Build history of the part. All positions in model axes, mm. A direction names the side the tool comes from. Coordinates: 2 decimals unless noted, no trailing zeros. Write each loop counter-clockwise with the first axis right and the second up, starting at its lowest first coordinate (ties: lowest second). Pieces come first, ordered by that corner, then holes. Notation, with made-up numbers: (-34, -2.75) -> (17, -2.75) arc R21 ccw to (17, 10.25) -> close; hole circle Ø10 at (-6.75, 24). An arc over 180 degrees is marked (long way). Write each question's results on one line, items separated by ' | '. Start each with the question number.
Q1. Saw through at C-C on x = 3. Give the cut face in (y, z), and give its area (3 significant figures).
Q2. Saw through at B-B on y = 4.5. Give the cut face in (x, z), and give its area (3 significant figures).
Q3. Saw through at D-D on z = 4.1. Give the cut face in (x, y).
Q4. Tool access for faces 1 (the face through (-3, -3.5, 2)), 2 (the face through (-3.75, 2.23, 2.54)), 3 (the face through (3.5, 3, 2)), 4 (the face through (3, -3.5, 2)): list every direction of +Z, -Z, +X, -X, +Y, -Y with a clear straight run to the whole face (end or side of a thin tool).
Q5. Saw through at A-A on z = 2.25. Give the cut face in (x, y), and give its area (3 significant figures).
Q6. Drill centre lines: line 1 (Y direction, x = -3.65, z = 2.25); line 2 (X direction, y = -3.75, z = 0.55); line 3 (X direction, y = -3, z = 0.3). Where is each one in solid material? Low to high.
Q7. Drop flat-ended pins along their axis: pin 1 Ø1 at (y, z) = (3, 1.5) entering from +X; pin 2 Ø0.5 at (x, z) = (3, 2) entering from -Y; pin 3 Ø0.8 at (y, z) = (4.5, 1.5) entering from +X. Give the stop position or say it passes through.
from build123d import *

# Parameters (mm, degrees)
SKETCH_4_W          = 5
SKETCH_4_H          = 10
EXTRUDE_2_DEPTH     = 4.5
SKETCH_5_W          = 4.5
SKETCH_5_H          = 7
EXTRUDE_3_DEPTH     = 1
SKETCH_6_W          = 4.5
SKETCH_6_H          = 7
EXTRUDE_4_DEPTH     = 1
SKETCH_7_R          = 2.25
EXTRUDE_5_DEPTH     = 0.5
SKETCH_8_R          = 0.25
CUT_EXTRUDE_1_DEPTH = 0.5
CUT_EXTRUDE_START   = -0.5
SKETCH_9_R          = 0.25
CUT_EXTRUDE_2_DEPTH = 0.5


with BuildPart() as part:
    # 草图4 → 凸台-拉伸2 (new body)
    with BuildSketch(Plane.XY):
        Rectangle(SKETCH_4_W, SKETCH_4_H)
    extrude(amount=EXTRUDE_2_DEPTH)

    # 草图5 → 凸台-拉伸3 (add)
    with BuildSketch(Plane(origin=(2.5, 0, 0), x_dir=(0, 0, -1), z_dir=(1, 0, 0))):
        with Locations((-2.25, 0)):
            Rectangle(SKETCH_5_W, SKETCH_5_H)
    extrude(amount=EXTRUDE_3_DEPTH)

    # 草图6 → 凸台-拉伸4 (add)
    with BuildSketch(Plane.ZY.offset(2.5)):
        with Locations((2.25, 0)):
            Rectangle(SKETCH_6_W, SKETCH_6_H)
    extrude(amount=EXTRUDE_4_DEPTH)

    # 草图7 → 凸台-拉伸5 (add)
    with BuildSketch(Plane(origin=(3.5, 0, 0), x_dir=(0, 0, -1), z_dir=(1, 0, 0))):
        with Locations((-2.25, 0)):
            Circle(SKETCH_7_R)
    extrude_5 = extrude(amount=EXTRUDE_5_DEPTH)

    # 镜向1: 凸台-拉伸5 across plane
    add(extrude_5.mirror(Plane(origin=(0, 0, 0), x_dir=(0, 0, 1), z_dir=(1, 0, 0))))

    # 草图8 → 切除-拉伸1 (cut)
    with BuildSketch(Plane(origin=(4, 0, 0), x_dir=(0, 0, -1), z_dir=(1, 0, 0))):
        with Locations((-2.25, 0)):
            Circle(SKETCH_8_R)
    extrude(amount=-CUT_EXTRUDE_1_DEPTH, mode=Mode.SUBTRACT)

    # 草图9 → 切除-拉伸2 (cut)
    with BuildSketch(Plane.ZY.offset(4).offset(CUT_EXTRUDE_START)):
        with Locations(Location((2.25, 0, 0), (0, 0, 180))):
            Circle(SKETCH_9_R)
    extrude(amount=CUT_EXTRUDE_2_DEPTH, mode=Mode.SUBTRACT)


solid = part.part
Returned:
1) outline: (-3.5, 0) -> (3.5, 0) -> (3.5, 4.5) -> (-3.5, 4.5) -> close | area: 31.5 mm2
2) outline: (-2.5, 0) -> (2.5, 0) -> (2.5, 4.5) -> (-2.5, 4.5) -> close | area: 22.5 mm2
3) outline: (-4, -1.28) -> (-3.5, -1.28) -> (-3.5, -3.5) -> (-2.5, -3.5) -> (-2.5, -5) -> (2.5, -5) -> (2.5, -3.5) -> (3.5, -3.5) -> (3.5, -1.28) -> (4, -1.28) -> (4, 1.28) -> (3.5, 1.28) -> (3.5, 3.5) -> (2.5, 3.5) -> (2.5, 5) -> (-2.5, 5) -> (-2.5, 3.5) -> (-3.5, 3.5) -> (-3.5, 1.28) -> (-4, 1.28) -> close
4) face 1: +Z, -Z, -X, -Y | face 2: -X | face 3: +X, +Y | face 4: +Z, -Z, +X, -Y
5) outline: (-4, -2.25) -> (-3.5, -2.25) -> (-3.5, -3.5) -> (-2.5, -3.5) -> (-2.5, -5) -> (2.5, -5) -> (2.5, -3.5) -> (3.5, -3.5) -> (3.5, -2.25) -> (4, -2.25) -> (4, -0.25) -> (3.5, -0.25) -> (3.5, 0.25) -> (4, 0.25) -> (4, 2.25) -> (3.5, 2.25) -> (3.5, 3.5) -> (2.5, 3.5) -> (2.5, 5) -> (-2.5, 5) -> (-2.5, 3.5) -> (-3.5, 3.5) -> (-3.5, 2.25) -> (-4, 2.25) -> (-4, 0.25) -> (-3.5, 0.25) -> (-3.5, -0.25) -> (-4, -0.25) -> close | area: 68.0 mm2
6) line 1: y = -2.25 to -0.25, 0.25 to 2.25 | line 2: x = -2.5 to 2.5 | line 3: x = -3.5 to 3.5
7) pin 1: stops at x = 3.5 | pin 2: stops at y = -3.5 | pin 3: stops at x = 2.5
